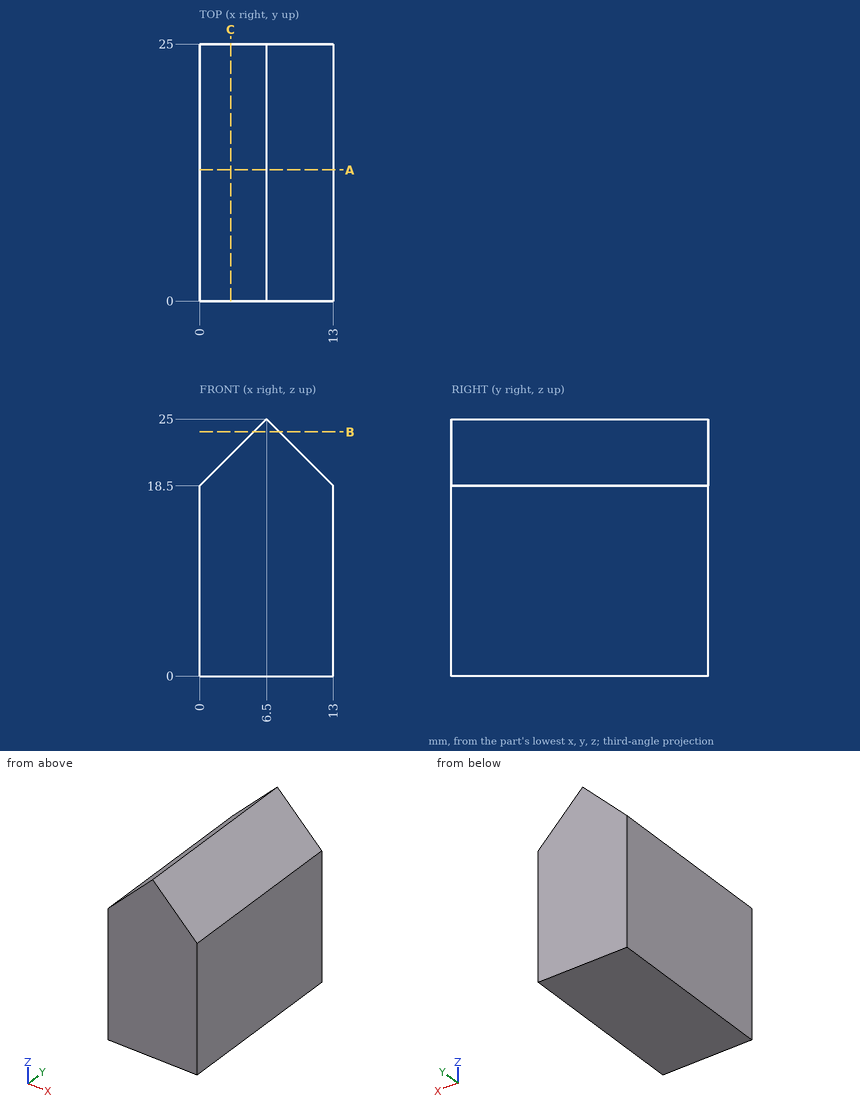
Answer from the drawing. Dimensions are ordinates in mm from the lowest x, y and z of the part. Round coordinates to 2 decimals unless told otherwise and drop trailing zeros. Loops run counter-clockwise (first coordinate to the right, second up) from the corner with the lowest first, then second, coordinate; pieces in that order, holes last.
1) Consider line 1 (Z direction, x = 12.25, y = 22.25); line 2 (Z direction, x = 5.5, y = 18.5); line 3 (X direction, y = 1.5, z = 22.75). Determine where each line is inside the solid, lowest interval first.
Outcome:
line 1: z = 0 to 19.25
line 2: z = 0 to 24
line 3: x = 4.25 to 8.75
2) A cutting plane is placed at A-A on y = 12.75. Determine the outline of the cut face in (x, z), plus the area to 3 significant figures.
Outcome:
outline: (0, 0) - (13, 0) - (13, 18.5) - (6.5, 25) - (0, 18.5) - close
area: 283 mm2
3) Given P1, Ø3, axis at x = 11, y = 13, coming from the +Z side; P2, Ø2, axis at y = 12, z = 22.5, coming from the -X side, each flat-ended and moving along its own axis, determine where each tip first touches the part or whether it passes through.
Outcome:
P1: stops at z = 22
P2: stops at x = 3
4) A cutting plane is placed at B-B on z = 23.75. Determine the outline of the cut face in (x, y).
Outcome:
outline: (5.25, 0) - (7.75, 0) - (7.75, 25) - (5.25, 25) - close
5) A cutting plane is placed at C-C on x = 3. Determine the outline of the cut face in (y, z), plus the area to 4 significant figures.
Outcome:
outline: (0, 0) - (25, 0) - (25, 21.5) - (0, 21.5) - close
area: 537.5 mm2
